Part model, mm, in its own coordinate system. Round coordinates to 2 decimals unless told otherwise and drop trailing zeros. Write each loop counter-clockwise with the first axis right and the second up, starting at its lowest first coordinate (ties: lowest second). Pieces come first, ordered by that corner, then holes. Notation, with made-up numbers: (28, 85) -> (73, 85) arc R19 ccw to (73, 93) -> close; hole circle Ø5 at (75.5, 5.25). An arc over 180 degrees is marked (long way). Return JSON: item names as keys, results as strings. Group by question number.
```python
from build123d import *

# Parameters (mm, degrees)
SKETCH1_R           = 12.5
CORPO_25_1056_DEPTH = 528
CHANFRO_1_45_SIZE   = 1


with BuildPart() as part:
    # Sketch1 → Corpo Ø25×1056 (new, symmetric)
    with BuildSketch(Plane.XY):
        Circle(SKETCH1_R)
    extrude(amount=CORPO_25_1056_DEPTH, both=True)

    # Sketch4 → Furo de Centro (revolve, cut)
    with BuildSketch(Plane(origin=(0, 0, -528), x_dir=(0, 1, 0), z_dir=(1, 0, 0))):
        Polygon((0, 0), (0, 10), (1.7, 8.978536948), (1.7, 2.511473671), (3.15, 0), align=None)
    furo_de_centro = revolve(axis=Axis((0, 0, -534.35), (0, 0, 1)), mode=Mode.SUBTRACT)

    # Furo de Centro Espelhado: Furo de Centro across plane
    add(furo_de_centro.mirror(Plane.XY), mode=Mode.SUBTRACT)

    # Chanfro 1×45°
    chanfro_1_45_edges = [part.edges().sort_by_distance(p)[0] for p in [
        (-12.5, 0, -528),
        (-12.5, 0, 528),
    ]]
    chamfer(chanfro_1_45_edges, length=CHANFRO_1_45_SIZE)


solid = part.part
```
Item 1: Flat gauge pins, fed straight in: P1, Ø4.5, axis at x = 0, y = 0, coming from the -Z side; P2, Ø1.5, axis at x = 3.5, z = -143, coming from the +Y side; P3, Ø3, axis at x = 8, z = 177.5, coming from the -Y side. Where does each tip first touch, or does it go through?
Item 2: Cut at A-A (z = -171.5). Write the cut outline in (x, y), then the cut area to 3 significant figures.
Item 3: Wall check: L1, parallel to Y at x = 0, z = 522; L2, parallel to Y at x = 0.75, z = 106; L3, parallel to X at y = 1.75, z = -270. Give the ranges that are in metal, low to high.
Checks:
{
 "1": {"P1": "stops at z = -526.44", "P2": "stops at y = 12.19", "P3": "stops at y = -10.68"},
 "2": {"outline": "circle Ø25 at (0, 0)", "area": "491 mm2"},
 "3": {"L1": "y = -12.5 to -1.7, 1.7 to 12.5", "L2": "y = -12.48 to 12.48", "L3": "x = -12.38 to 12.38"}
}
